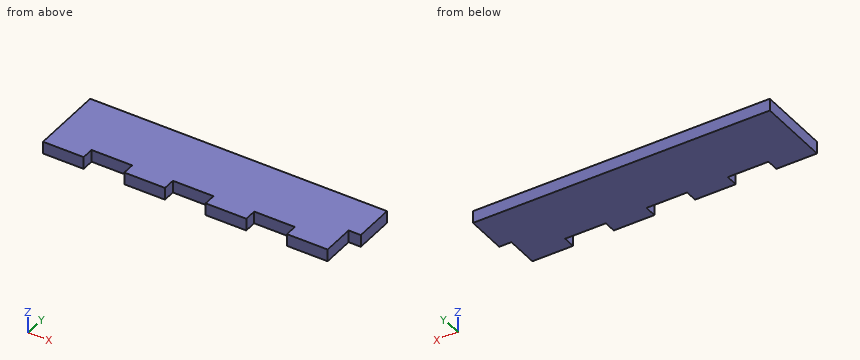
from build123d import *

# Parameters (mm, degrees)
ESQUISSE1_W                = 70
ESQUISSE1_H                = 18
BOSS_EXTRU_1_DEPTH         = 3
ESQUISSE2_W                = 10
ESQUISSE2_H                = 3
ENL_V_MAT_EXTRU_1_DEPTH    = 3
R_P_TITION_LIN_AIRE1_COUNT = 3
R_P_TITION_LIN_AIRE1_PITCH = 20
ESQUISSE3_W                = 3
ESQUISSE3_H                = 10
BOSS_EXTRU_2_DEPTH         = 3


with BuildPart() as part:
    # Esquisse1 → Boss.-Extru.1 (new body)
    with BuildSketch(Plane.XY):
        with Locations((35, -9)):
            Rectangle(ESQUISSE1_W, ESQUISSE1_H)
    extrude(amount=BOSS_EXTRU_1_DEPTH)

    # Esquisse2 → Enlèv. mat.-Extru.1 (cut)
    with BuildSketch(Plane.XY.offset(3)):
        with Locations((55, -16.5)):
            Rectangle(ESQUISSE2_W, ESQUISSE2_H)
    enl_v_mat_extru_1 = extrude(amount=-ENL_V_MAT_EXTRU_1_DEPTH, mode=Mode.SUBTRACT)

    # Répétition linéaire1: Enlèv. mat.-Extru.1 ×3
    with Locations(*[(-i * R_P_TITION_LIN_AIRE1_PITCH, 0, 0) for i in range(1, R_P_TITION_LIN_AIRE1_COUNT)]):
        add(enl_v_mat_extru_1, mode=Mode.SUBTRACT)

    # Esquisse3 → Boss.-Extru.2 (add)
    with BuildSketch(Plane(origin=(70, 0, 0), x_dir=(0, 0, -1), z_dir=(1, 0, 0))):
        with Locations((-1.5, -5)):
            Rectangle(ESQUISSE3_W, ESQUISSE3_H)
    extrude(amount=BOSS_EXTRU_2_DEPTH)


solid = part.part
Work out the finished part from the listing and answer in its coordinate system (mm). Coordinates: 2 decimals unless noted, no trailing zeros. Write each loop counter-clockwise with the first axis right and the second up, starting at its lowest first coordinate (ties: lowest second). Pieces come first, ordered by that corner, then holes.
1. The part is cut by section C-C, the plane x = 56. Write down the section's boundary in (y, z), and give its area (3 significant figures).
Results list:
outline: (-15, 0) - (0, 0) - (0, 3) - (-15, 3) - close
area: 45.0 mm2
2. The part is cut by section A-A, the plane z = 0.95. Write down the section's boundary in (x, y).
Results list:
outline: (0, -18) - (10, -18) - (10, -15) - (20, -15) - (20, -18) - (30, -18) - (30, -15) - (40, -15) - (40, -18) - (50, -18) - (50, -15) - (60, -15) - (60, -18) - (70, -18) - (70, -10) - (73, -10) - (73, 0) - (0, 0) - close
3. The part is cut by section B-B, the plane y = -10.75. Write down the section's boundary in (x, z).
Results list:
outline: (0, 0) - (70, 0) - (70, 3) - (0, 3) - close
4. Consider line 1 along X through (y, z) = (-16, 2.45); line 2 along X through (y, z) = (-10.5, 1.45); line 3 along Y through (x, z) = (54.5, 0.45). Determine where each line is inside the solid, lowest interval first.
Results list:
line 1: x = 0 to 10, 20 to 30, 40 to 50, 60 to 70
line 2: x = 0 to 70
line 3: y = -15 to 0
5. Flat-ended cylindrical pins translate along their axes: pin 1 (1.5 mm diameter, centred on y = -15, z = 2, fed in from +X); pin 2 (0.9 mm diameter, centred on x = 71, z = 1, fed in from -Y); pin 3 (1.5 mm diameter, centred on x = 54.5, z = 1.5, fed in from -Y). Find the tip coordinate at first contact, or state that the pin passes through.
Results list:
pin 1: stops at x = 70
pin 2: stops at y = -10
pin 3: stops at y = -15
